Check sheet for the drawn part. Datum: minimum x, y, z corner. Units: mm. A direction names the side the tool comes from. Give positions to 0.01 mm unless a question says otherwise; leave off trailing zeros. Order: outer loops, then holes, each group sorted by start corner. A loop starts at its lowest first (then second) coordinate and runs counter-clockwise, first axis right, second up. Notation, with made-up numbers: M 84.25,18 L 139.25,18 A18 cw 139.25,29 Z; hole C 22.25,54 d3. An arc over 180 degrees is marked long. One line per question, with ' | ' between items. Start each with the question number.
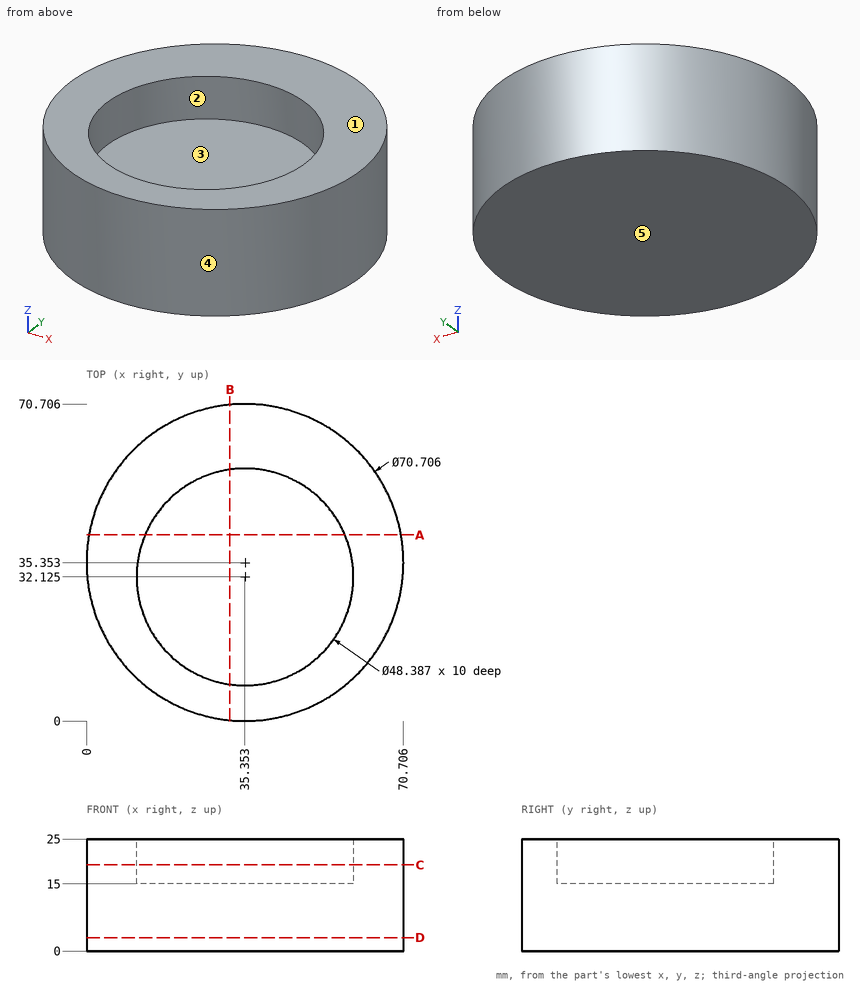
Item 1: Set-up check for the marked faces 1 and 2: record each of +Z, -Z, +X, -X, +Y, -Y from which the full face is reachable in a straight line by a thin tool's end or side.
Item 2: Scan lines: probe 1 along Z at (x, y) = (30.5, 44); probe 2 along X at (y, z) = (44.5, 17.5) (1 decimal); probe 3 along Y at (x, z) = (50, 15.5) (1 decimal). Record each from-to range of solid material in increasing order. Write a range as [from, to].
Item 3: Go/stop test with flat-tipped pins: P1, Ø4, axis at x = 56, y = 40.5, coming from the -Z side; P2, Ø1, axis at y = 14, z = 17.5, coming from the +X side; P3, Ø5, axis at y = 25, z = 20, coming from the -X side; P4, Ø10, axis at x = 56.5, z = 7, coming from the -Y side. Record where each tip stops, or that it passes through.
Item 4: Section check D-D, the plane z = 3. Record the cut outline in (x, y).
Item 5: Section check C-C, the plane z = 19.25. Record the cut outline in (x, y) (1 decimal).
Item 6: Draft check along Y on the marked faces 3, 4 and 5. Enter one of: released by +Y, released by -Y, zero draft, split by the parting line, or undercut.
Item 7: Section check A-A, the plane y = 41.5. Record the cut outline in (x, z), then the cut area to 3 significant figures.
Item 8: Section check B-B, the plane x = 32. Record the cut outline in (y, z) (1 decimal).
Reported:
1) face 1: +Z, +X, -X, +Y, -Y | face 2: +Z
2) probe 1: z = [0, 15] | probe 2: x = [1.2, 14.6], [56.1, 69.5] | probe 3: y = [3.2, 12.9], [51.4, 67.5]
3) P1: stops at z = 0 | P2: stops at x = 63.9 | P3: stops at x = 0.88 | P4: stops at y = 3.9
4) outline: C 35.35,35.35 d70.71
5) outline: C 35.4,35.4 d70.7; hole C 35.4,32.1 d48.4
6) face 3: undercut | face 4: split by the parting line | face 5: zero draft
7) outline: M 0.54,0 L 70.17,0 L 70.17,25 L 57.66,25 L 57.66,15 L 13.05,15 L 13.05,25 L 0.54,25 Z | area: 1,290 mm^2
8) outline: M 0.2,0 L 70.5,0 L 70.5,25 L 56.1,25 L 56.1,15 L 8.2,15 L 8.2,25 L 0.2,25 Z
